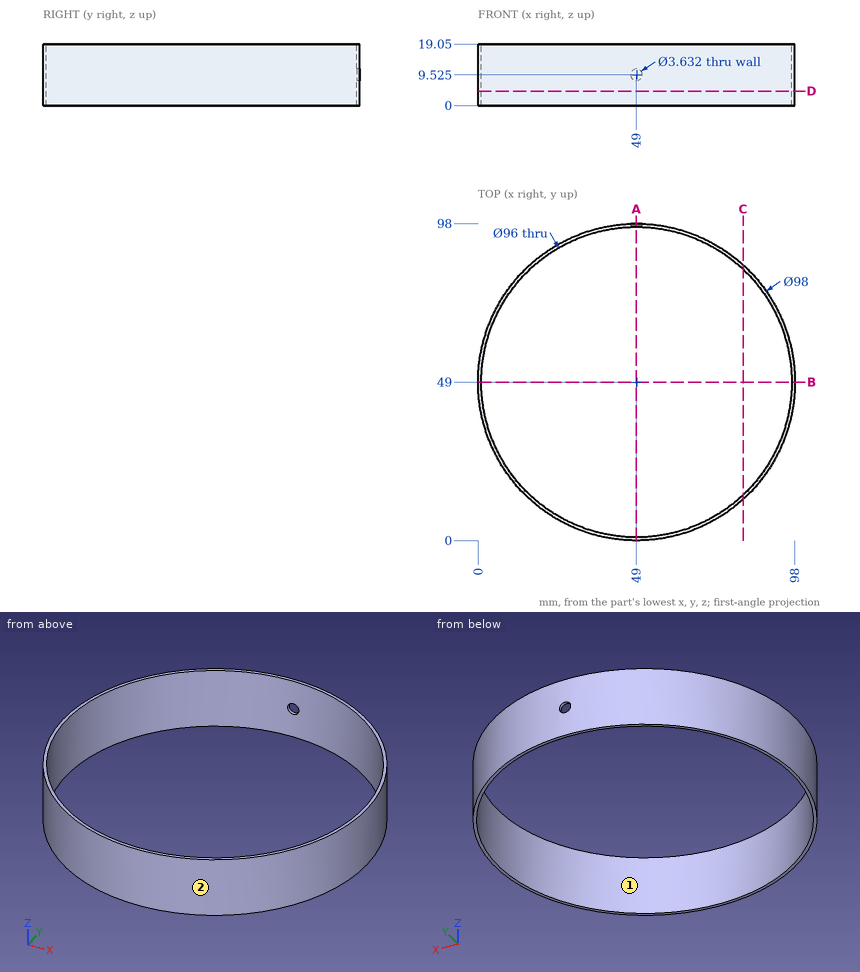
Here's the drawing with two shaded views (mm, measured from the low corner). I have some questions. Coordinates: 2 decimals unless noted, no trailing zeros. Order: outer loops, then holes, each group sorted by start corner. A loop starts at its lowest first (then second) coordinate and runs counter-clockwise, first axis right, second up.
Q1. Please list where these lines run through material, in increasing order: L1, parallel to X at y = 47.5, z = 18.25; L2, parallel to Z at x = 49, y = 97.7; L3, parallel to X at y = 9, z = 8.
Q2. Suppose I cut it at B-B on y = 49. Please give me the cut outline in (x, z).
Q3. Suppose I cut it at D-D on z = 4.5. Please give me the cut outline in (x, y).
Q4. Suppose I cut it at C-C on x = 82. Please give me the cut outline in (y, z).
Q5. Thinking about a two-plate mould opening in Y: for the marked faces 1 and 2, which applies, released by +Y, released by -Y, zero draft, split by the parting line, or undercut?
Q6. Will these pins go through, and if not, where does the flat tip stop? pin 1 (1.5 mm diameter, centred on y = 38, z = 16, fed in from +X); pin 2 (3 mm diameter, centred on y = 11, z = 4, fed in from +X); pin 3 (8 mm diameter, centred on y = 25, z = 15.5, fed in from -X); pin 4 (10 mm diameter, centred on x = 84, y = 33.5, fed in from -Z).
Q7. Suppose I cut it at A-A on x = 49. Please give me the cut outline in (y, z).
Answer:
1. L1: x = 0.02 to 1.02, 96.98 to 97.98
1. L2: z = 0 to 7.71, 11.34 to 19.05
1. L3: x = 20.7 to 22.47, 75.53 to 77.3
2. outline: (0, 0) - (1, 0) - (1, 19.05) - (0, 19.05) - close; (97, 0) - (98, 0) - (98, 19.05) - (97, 19.05) - close
3. outline: circle Ø98 at (49, 49); hole circle Ø96 at (49, 49)
4. outline: (12.78, 0) - (14.14, 0) - (14.14, 19.05) - (12.78, 19.05) - close; (83.86, 0) - (85.22, 0) - (85.22, 19.05) - (83.86, 19.05) - close
5. face 1: undercut
5. face 2: split by the parting line
6. pin 1: stops at x = 96.92
6. pin 2: stops at x = 81.69
6. pin 3: stops at x = 4.27
6. pin 4: passes through
7. outline: (0, 0) - (1, 0) - (1, 19.05) - (0, 19.05) - close; (97, 0) - (98, 0) - (98, 7.71) - (97, 7.71) - close; (97, 11.34) - (98, 11.34) - (98, 19.05) - (97, 19.05) - close
